Design review of the part built by this model. Coordinates are the model's own, in mm. Round coordinates to 2 decimals unless told otherwise and drop trailing zeros. Loops run counter-clockwise (first coordinate to the right, second up) from the corner with the lowest first, then second, coordinate; pieces in that order, holes last. Notation, with made-up numbers: (32.25, 67) - (51.25, 67) arc R18 ccw to (51.25, 71) - close; hole circle Ø8 at (49, -9). An arc over 180 degrees is marked (long way). Use one line per item in the form item = value. Start each with the question number.
(1) We need section D-D, the plane x = -2.25. Write out the cut boundary in (y, z), then the cut area to 3 significant figures.
(2) We need section C-C, the plane y = -2. Write out the cut boundary in (x, z).
(3) We need section A-A, the plane x = 0. Write out the cut boundary in (y, z).
(4) We need section B-B, the plane z = 0. Write out the cut boundary in (x, y).
(5) For pin 1 (1 mm diameter, centred on y = -1.5, z = -0.5, fed in from -X); pin 2 (1 mm diameter, centred on y = 2, z = -1, fed in from -X); pin 3 (3.5 mm diameter, centred on x = 0, z = 0, fed in from +Y), all flat-tipped, find the tip position at first contact; note any pin that passes through.
(6) Wall thickness on probe 1 along Y at (x, z) = (-2, -1.5); probe 2 along X at (y, z) = (1.75, -0.25); probe 3 along X at (y, z) = (-2.25, -1): over which ranges is each line inside the solid? List them lowest first. Write a range as [from, to].
(7) The part is to be moulded in two halves that separate along Z. For faces 1 (the flat face through (2, 3, 0)), 2 (the cylindrical face through (1.5, 0.04, 0.07)), say which applies: released by +Z, released by -Z, zero draft, split by the parting line, or undercut.
Autodesk Inventor part; units mm, degrees
ref_plane "YZ Plane" through (0, 0, 0) normal (1, 0, 0) x (0, 1, 0)
ref_plane "XZ Plane" through (0, 0, 0) normal (0, 1, 0) x (-1, 0, 0)
ref_plane "XY Plane" through (0, 0, 0) normal (0, 0, 1) x (1, 0, 0)
sketch "Эскиз1" plane through (0, 0, 0) normal (0, 1, 0) x (-1, 0, 0)
  circle A0 centre (0, 0) radius 3.969
  line L0 (3.969, 0) -> (-3.969, 0)
  dimension "d0" = 7.938
  dimension "d1" = 7.938
revolve "Вращение1" add sketch "Эскиз1" angle 360 about axis through (-3.969, 0, 0) along (1, 0, 0) picked at (1.323, -1.2297) contours A0 L0
sketch "Эскиз2" plane through (0, 0, 0) normal (0, 1, 0) x (-1, 0, 0)
  circle A0 centre (0, 0) radius 1.5
  dimension "d3" = 3
extrude "Выдавливание1" cut sketch "Эскиз2" along normal mid plane 10
sketch "Эскиз3" plane through (0, 0, 0) normal (1, 0, 0) x (0, 1, 0)
  line L0 (13, 10) -> (3, 10)
  line L1 (3, 10) -> (3, -10)
  line L2 (3, -10) -> (13, -10)
  line L3 (13, -10) -> (13, 10)
  point P0 (0, 0)
  dimension "d6" = 3
  dimension "d7" = 20
  dimension "d8" = 10
  dimension "d9" = 10
extrude "Выдавливание2" cut sketch "Эскиз3" along normal through all both and the other way through all
mirror "Зеркальное отражение1" about plane through (0, 0, 0) normal (0, 1, 0) of "Выдавливание2"
properties part number "Ball" material "Нержавеющая сталь"
Data:
q1.outline = (-3, -1.3) arc R3.27 ccw to (3, -1.3) - (3, 1.3) arc R3.27 ccw to (-3, 1.3) - close
q1.area = 32.6 mm^2
q2.outline = circle Ø6.86 at (0, 0); hole circle Ø3 at (0, 0)
q3.outline = (-3, -2.6) arc R3.97 ccw to (3, -2.6) - (3, -1.5) - (-3, -1.5) - close; (-3, 1.5) - (3, 1.5) - (3, 2.6) arc R3.97 ccw to (-3, 2.6) - close
q4.outline = (-2.6, -3) - (-1.5, -3) - (-1.5, 3) - (-2.6, 3) arc R3.97 ccw to start; (1.5, -3) - (2.6, -3) arc R3.97 ccw to (2.6, 3) - (1.5, 3) - close
q5.pin_1 = -3.82
q5.pin_2 = -3.57
q5.pin_3 = 3
q6.probe_1 = [-3, 3]
q6.probe_2 = [-3.55, -1.48], [1.48, 3.55]
q6.probe_3 = [-3.11, -1.12], [1.12, 3.11]
q7.face_1 = zero draft
q7.face_2 = undercut
